from build123d import *
from build123d.topology import SkipClean

# Parameters (mm, degrees)
MODEL_R             = 1
MODEL_R_2           = 1.25
BOSS_EXTRUDE1_DEPTH = 30
SKETCH3_R           = 2.5
BOSS_EXTRUDE2_DEPTH = 30
BOSS_EXTRUDE5_START = 3
SKETCH7_R           = 2.5
SKETCH7_R_2         = 1
BOSS_EXTRUDE5_DEPTH = 3
BOSS_EXTRUDE6_DEPTH = 3


with BuildPart() as part:
    # Model → Boss-Extrude1 (new body)
    # profile 1 of 2: a face of its own
    with BuildSketch(Plane.XY):
        Polygon((25.100694962, 10.3343272), (45.100694962, 30.3343272), (50.757549212, 24.67747295), (30.757549212, 4.67747295), align=None)
        with Locations((41.464655993, 21.041433981)):
            Circle(MODEL_R, mode=Mode.SUBTRACT)
        with Locations((34.393588181, 13.970366169)):
            Circle(MODEL_R, mode=Mode.SUBTRACT)
    # profile 2 of 2: a face of its own
    with BuildSketch(Plane.XY):
        Polygon((40.100694962, 42.8343272), (45.100694962, 42.8343272), (45.100694962, 30.3343272), (25.100694962, 10.3343272), (12.600694962, 10.3343272), (12.600694962, 15.3343272), (23.02962715, 15.3343272), (40.100694962, 32.405395011), align=None)
        with Locations((33.332928009, 22.102094153)):
            Circle(MODEL_R_2, mode=Mode.SUBTRACT)
        with Locations((42.600694962, 37.8343272)):
            Circle(MODEL_R_2, mode=Mode.SUBTRACT)
        with Locations((17.600694962, 12.8343272)):
            Circle(MODEL_R_2, mode=Mode.SUBTRACT)
    extrude(amount=BOSS_EXTRUDE1_DEPTH)

    # Sketch3 → Boss-Extrude2 (add)
    with BuildSketch(Plane(origin=(0, 0, 0), x_dir=(-1, 0, 0), z_dir=(0, 0, -1))):
        Polygon((-30.757549212, 4.67747295), (-59.041820459, -23.606798297), (-65.40578149, -29.970759328), (-85.40578149, -9.970759328), (-79.041820459, -3.606798297), (-62.577354365, -20.071264391), (-34.293083118, 8.213006856), align=None)
        with Locations((-76.033069792, -12.979509995)):
            Circle(SKETCH3_R, mode=Mode.SUBTRACT)
        with Locations((-68.96200198, -20.050577807)):
            Circle(SKETCH3_R, mode=Mode.SUBTRACT)
    extrude(amount=-BOSS_EXTRUDE2_DEPTH)

    # Sketch7 → Boss-Extrude5 (add)
    with SkipClean():  # the faces are left unmerged after this step: merging them gives an invalid solid
        with BuildSketch(Plane(origin=(0, 0, 0), x_dir=(-1, 0, 0), z_dir=(0, 0, -1)).offset(BOSS_EXTRUDE5_START)):
            Polygon((-45.100694962, 30.3343272), (-25.100694962, 10.3343272), (-65.40578149, -29.970759328), (-85.40578149, -9.970759328), (-79.041820459, -3.606798297), (-62.577354365, -20.071264391), (-34.293083118, 8.213006856), (-50.757549212, 24.67747295), align=None)
            with Locations((-68.96200198, -20.050577807)):
                Circle(SKETCH7_R, mode=Mode.SUBTRACT)
            with Locations((-76.033069792, -12.979509995)):
                Circle(SKETCH7_R, mode=Mode.SUBTRACT)
            with Locations((-34.393588181, 13.970366169)):
                Circle(SKETCH7_R_2, mode=Mode.SUBTRACT)
            with Locations((-41.464655993, 21.041433981)):
                Circle(SKETCH7_R_2, mode=Mode.SUBTRACT)
        extrude(amount=-BOSS_EXTRUDE5_DEPTH)

    # Sketch8 → Boss-Extrude6 (add)
    with SkipClean():  # the faces are left unmerged after this step: merging them gives an invalid solid
        with BuildSketch(Plane(origin=(0, 0, -3), x_dir=(-1, 0, 0), z_dir=(0, 0, -1))):
            Polygon((-50.757549212, 24.67747295), (-34.293083118, 8.213006856), (-62.577354365, -20.071264391), (-79.041820459, -3.606798297), align=None)
        extrude(amount=-BOSS_EXTRUDE6_DEPTH)


solid = part.part
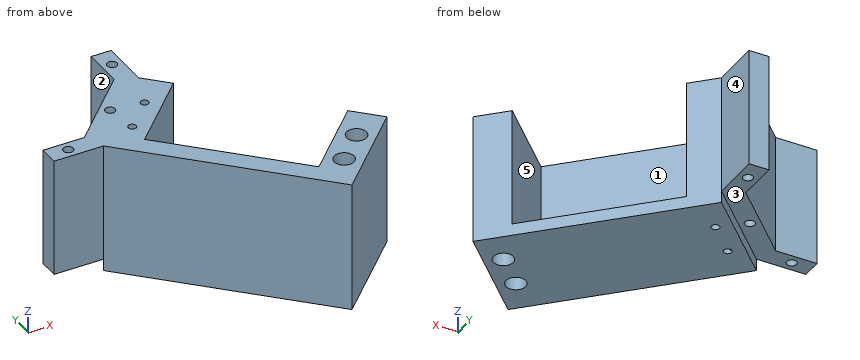
Can you work these out from the model? Positions are in its coordinate system, mm. Face numbers are marked on the shaded views. A direction names the side the tool comes from. Give positions to 0.01 mm unless a question says otherwise; leave off trailing zeros. Order: outer loops, then holes, each group sorted by start corner. A loop starts at its lowest first (then second) coordinate and runs counter-clockwise, first axis right, second up. Notation, with made-up numbers: M 36.5,70.25 L 51.5,70.25 A17 ccw 51.5,102.25 Z; hole C 80.5,84.5 d1. An arc over 180 degrees is marked long. Use one line per item in the form item = value.
Item 1: For the marked faces 1, 2, 3, 4 and 5, which set-ups out of +Z, -Z, +X, -X, +Y, -Y let a thin tool reach every point of the face, with its end or its side?
Values follow:
face_1 = +Z
face_2 = +Z, -Z, -X, +Y
face_3 = -Z, -X, +Y
face_4 = +Z, -Z, +X, +Y
face_5 = +Z, +Y
Item 2: If we section it at A-A, the plane z = 24: Write out the boundary of the cut face in (x, y).
Values follow:
outline = M 12.6,10.33 L 25.1,10.33 L 65.41,-29.97 L 85.41,-9.97 L 79.04,-3.61 L 62.58,-20.07 L 34.29,8.21 L 50.76,24.68 L 45.1,30.33 L 45.1,42.83 L 40.1,42.83 L 40.1,32.41 L 23.03,15.33 L 12.6,15.33 Z; hole C 17.6,12.83 d2.5; hole C 33.33,22.1 d2.5; hole C 34.39,13.97 d2; hole C 41.46,21.04 d2; hole C 42.6,37.83 d2.5; hole C 68.96,-20.05 d5; hole C 76.03,-12.98 d5
Item 3: If we section it at B-B, the plane x = 74.5: Write out the boundary of the cut face in (y, z), and give its area (3 significant figures).
Values follow:
outline = M -20.88,-3 L -14.95,-3 L -14.95,30 L -20.88,30 Z; M -11,-3 L 0.94,-3 L 0.94,0 L -8.15,0 L -8.15,30 L -11,30 Z
area = 317 mm^2
Item 4: If we section it at C-C, the plane x = 54: Write out the boundary of the cut face in (y, z).
Values follow:
outline = M -18.56,-3 L 21.44,-3 L 21.44,0 L -11.49,0 L -11.49,30 L -18.56,30 Z
Item 5: Will these pins go through, and if not, where does the flat tip stop? pin 1 Ø6 at (x, y) = (40.5, 33.5) entering from -Z; pin 2 Ø22.5 at (x, y) = (58, 8.5) entering from +Z; pin 3 Ø1 at (x, z) = (34.5, 19.5) entering from -Y (3 decimals).
Values follow:
pin_1 = 0
pin_2 = 0
pin_3 = 0.435
Item 6: If we section it at D-D, the plane y = -1.5: Write out the boundary of the cut face in (x, z).
Values follow:
outline = M 36.94,-3 L 76.94,-3 L 76.94,0 L 44.01,0 L 44.01,30 L 36.94,30 Z
Item 7: If I drill on line 1 along X through (y, z) = (-19.5, 5); line 2 along Y through (x, z) = (41.5, 20); line 3 along X through (y, z) = (35, 17), over which ranges is the centre line in solid material (lowest first)? Write a range as [from, to].
Values follow:
line_1 = [54.94, 62.01], [63.15, 66.52], [71.4, 75.88]
line_2 = [-6.06, 1.01], [15.42, 20.04], [22.04, 37.24], [38.43, 42.83]
line_3 = [40.1, 45.1]
